Input: dimensioned drawing with shaded views. Units: mm. Origin: part minimum x, y, z. A direction names the side the tool comes from. Give positions to 0.01 mm unless a question says otherwise; leave off trailing zeros. Loops run counter-clockwise (first coordinate to the right, second up) from the corner with the lowest first, then second, coordinate; pieces in that order, holes last.
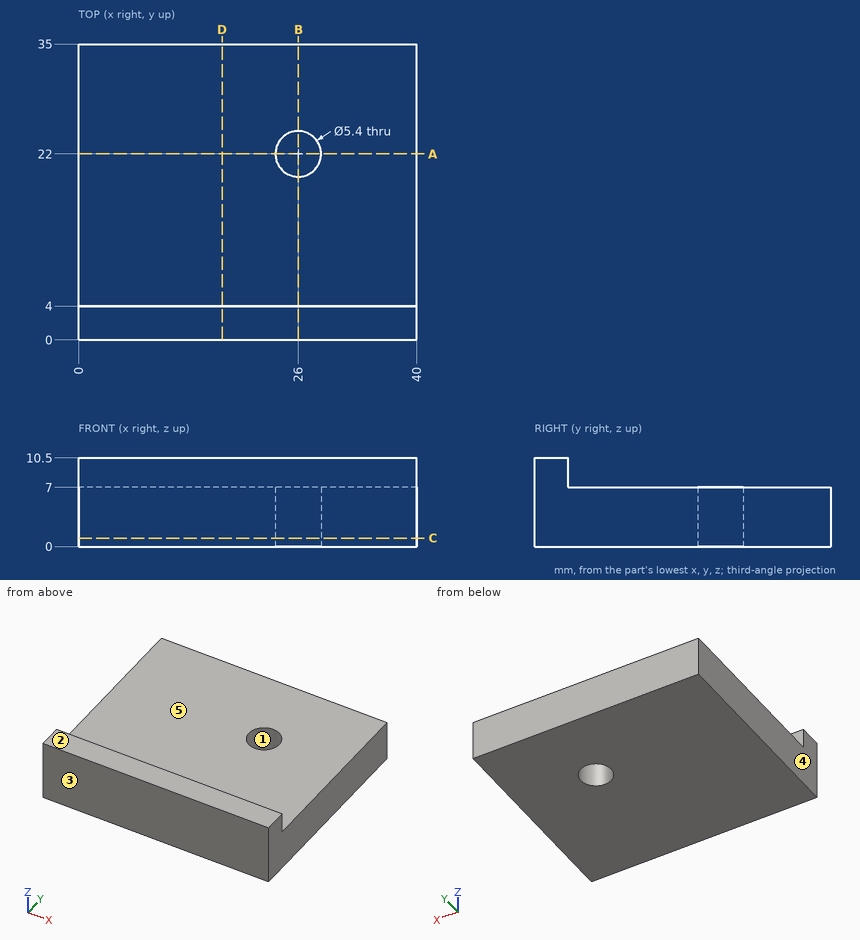
Item 1: Set-up query: the marked faces 4 and 5. Return all of +Z, -Z, +X, -X, +Y, -Y with unobstructed straight access to the full face (end or side cutting, diameter ignored); none if empty.
Values follow:
face 4: +Z, -Z, -X, +Y, -Y
face 5: +Z, +X, -X, +Y
Item 2: Section query A-A on y = 22. Return loops of the section in (x, z).
Values follow:
outline: (0, 0) - (23.3, 0) - (23.3, 7) - (0, 7) - close; (28.7, 0) - (40, 0) - (40, 7) - (28.7, 7) - close
Item 3: Section query C-C on z = 1. Return loops of the section in (x, y), plus the area to 3 significant figures.
Values follow:
outline: (0, 0) - (40, 0) - (40, 35) - (0, 35) - close; hole circle Ø5.4 at (26, 22)
area: 1,380 mm2
Item 4: Draft query along Y for the marked faces 1, 2 and 3. Return one class per face: +Y half, -Y half, draft (parallel to the pull), parting line (faces both ways), or undercut.
Values follow:
face 1: undercut
face 2: draft
face 3: -Y half
Item 5: Section query B-B on x = 26. Return loops of the section in (y, z).
Values follow:
outline: (0, 0) - (19.3, 0) - (19.3, 7) - (4, 7) - (4, 10.5) - (0, 10.5) - close; (24.7, 0) - (35, 0) - (35, 7) - (24.7, 7) - close
Item 6: Ray query, probe 1 along Y at (x, z) = (26, 3.25); probe 2 along Z at (x, y) = (17, 13.5); probe 3 along Y at (x, z) = (24.5, 3) (3 decimals). Return the intervals inside material, ascending.
Values follow:
probe 1: y = 0 to 19.3, 24.7 to 35
probe 2: z = 0 to 7
probe 3: y = 0 to 19.755, 24.245 to 35
Item 7: Section query D-D on x = 17. Return loops of the section in (y, z), plus the area to 3 significant figures.
Values follow:
outline: (0, 0) - (35, 0) - (35, 7) - (4, 7) - (4, 10.5) - (0, 10.5) - close
area: 259 mm2
Item 8: Pin query (flat end, axial travel): pin 1 (2 mm diameter, centred on x = 16, y = 18, fed in from +Z); pin 2 (3 mm diameter, centred on x = 26, y = 22, fed in from -Z); pin 3 (3 mm diameter, centred on x = 14, z = 9, fed in from +Y). Return the tip coordinate at first contact, or that it passes through.
Values follow:
pin 1: stops at z = 7
pin 2: passes through
pin 3: stops at y = 4
